Autodesk Inventor part; units mm, degrees
ref_plane "YZ Plane" through (0, 0, 0) normal (1, 0, 0) x (0, 1, 0)
ref_plane "XZ Plane" through (0, 0, 0) normal (0, 1, 0) x (-1, 0, 0)
ref_plane "XY Plane" through (0, 0, 0) normal (0, 0, 1) x (1, 0, 0)
sketch "Sketch1" plane through (0, 0, 0) normal (0, 0, 1) x (1, 0, 0)
  circle A0 centre (0, 0) radius 12.5
  circle A1 centre (-15.4996, 15.5) radius 1.5
  circle A2 centre (-15.5, -15.4996) radius 1.5
  circle A3 centre (15.4996, -15.5) radius 1.5
  circle A4 centre (15.5, 15.4996) radius 1.5
  circle A5 centre (-23.5679, 23.5679) radius 2.5
  circle A6 centre (-23.5679, -23.5679) radius 2.5
  circle A7 centre (23.5679, -23.5679) radius 2.5
  circle A8 centre (23.5679, 23.5679) radius 2.5
  line L0 (0, 0) -> (-27.3582, 27.3582) construction
  line L1 (-32, 30) -> (32, 30)
  line L2 (32, 30) -> (32, -30)
  line L3 (32, -30) -> (-32, -30)
  line L4 (-32, -30) -> (-32, 30)
  dimension "d0" = 3
  dimension "d1" = 21.92
  dimension "d4" = 360
  dimension "d6" = 15.5
  dimension "d7" = 25
  dimension "d8" = 5
  dimension "d9" = 33.33
  dimension "d12" = 360
  dimension "d14" = 0
  dimension "d15" = 64
  dimension "d16" = 60
  dimension "d17" = 30
  dimension "d18" = 32
extrude "Extrusion1" add sketch "Sketch1" along normal blind 8
sketch "Sketch2" plane through (0, 0, 8) normal (0, 0, 1) x (1, 0, 0)
  line L0 (-21.5, 21.5) -> (21.5, 21.5)
  line L1 (21.5, 21.5) -> (21.5, -21.5)
  line L2 (21.5, -21.5) -> (-21.5, -21.5)
  line L3 (-21.5, -21.5) -> (-21.5, 21.5)
  point P0 (0, 0)
  dimension "d21" = 43
  dimension "d22" = 43
  dimension "d23" = 21.5
  dimension "d24" = 21.5
extrude "Extrusion2" cut sketch "Sketch2" against normal blind 4
fillet "Fillet1" radius 3 4 edges at (32, 30, 4) (-32, 30, 4) (-32, -30, 4) (32, -30, 4)
equation "\"d21\" = d22"
properties part number "motor support"
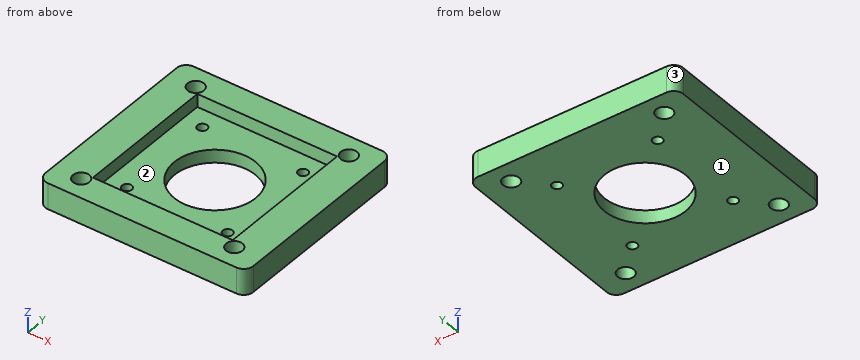
Part model, mm, in its own coordinate system. Face numbers are marked on the shaded views. Round coordinates to 2 decimals unless told otherwise and drop trailing zeros. Write each loop counter-clockwise with the first axis right and the second up, starting at its lowest first coordinate (ties: lowest second). Pieces come first, ordered by that corner, then holes. Notation, with made-up numbers: M 76.5,66.25 L 98.5,66.25 A12 cw 98.5,88.25 Z; hole C 79,51.25 d10. An arc over 180 degrees is marked long. Return JSON: item names as keys, results as strings. Group by question number.
(1) Pin check, flat tip, straight feed: pin 1 Ø1.8 at (x, y) = (15.5, 15.5) entering from +Z. Stop position of the tip, or through.
(2) Saw through at B-B on x = 0. Write the cut outline in (y, z), then the cut area to 3 significant figures.
(3) Two-plate mould, pull along X, no slides. Class the marked faces 1, 2 and 3: +X half, -X half, draft (parallel to the pull), parting line (faces both ways), or undercut.
(4) Saw through at D-D on z = 5. Write the cut outline in (x, y).
(5) Drill centre lines: probe 1 along Y at (x, z) = (15.5, 2.55); probe 2 along X at (y, z) = (-15.5, 2.7); probe 3 along Y at (x, z) = (-14.5, 4.75). Where is each one in solid material? Low to high.
(6) Saw through at C-C on y = 9.5. Write the cut outline in (x, z), then the cut area to 3 significant figures.
(7) Saw through at A-A on x = 15.5. Write the cut outline in (y, z), then the cut area to 3 significant figures.
Returned:
{
 "1": {"pin 1": "through"},
 "2": {"outline": "M -30,0 L -12.5,0 L -12.5,4 L -21.5,4 L -21.5,8 L -30,8 Z; M 12.5,0 L 30,0 L 30,8 L 21.5,8 L 21.5,4 L 12.5,4 Z", "area": "208 mm²"},
 "3": {"face 1": "draft", "face 2": "undercut", "face 3": "-X half"},
 "4": {"outline": "M -32,-27 A3 ccw -29,-30 L 29,-30 A3 ccw 32,-27 L 32,27 A3 ccw 29,30 L -29,30 A3 ccw -32,27 Z; hole C -23.57,-23.57 d5; hole C -23.57,23.57 d5; hole M -21.5,-21.5 L 21.5,-21.5 L 21.5,21.5 L -21.5,21.5 Z; hole C 23.57,-23.57 d5; hole C 23.57,23.57 d5"},
 "5": {"probe 1": "-30 to -17, -14 to 14, 17 to 30", "probe 2": "-32 to -17, -14 to 14, 17 to 32", "probe 3": "-30 to -21.5, 21.5 to 30"},
 "6": {"outline": "M -32,0 L -8.12,0 L -8.12,4 L -21.5,4 L -21.5,8 L -32,8 Z; M 8.12,0 L 32,0 L 32,8 L 21.5,8 L 21.5,4 L 8.12,4 Z", "area": "275 mm²"},
 "7": {"outline": "M -30,0 L -17,0 L -17,4 L -21.5,4 L -21.5,8 L -30,8 Z; M -14,0 L 14,0 L 14,4 L -14,4 Z; M 17,0 L 30,0 L 30,8 L 21.5,8 L 21.5,4 L 17,4 Z", "area": "284 mm²"}
}
